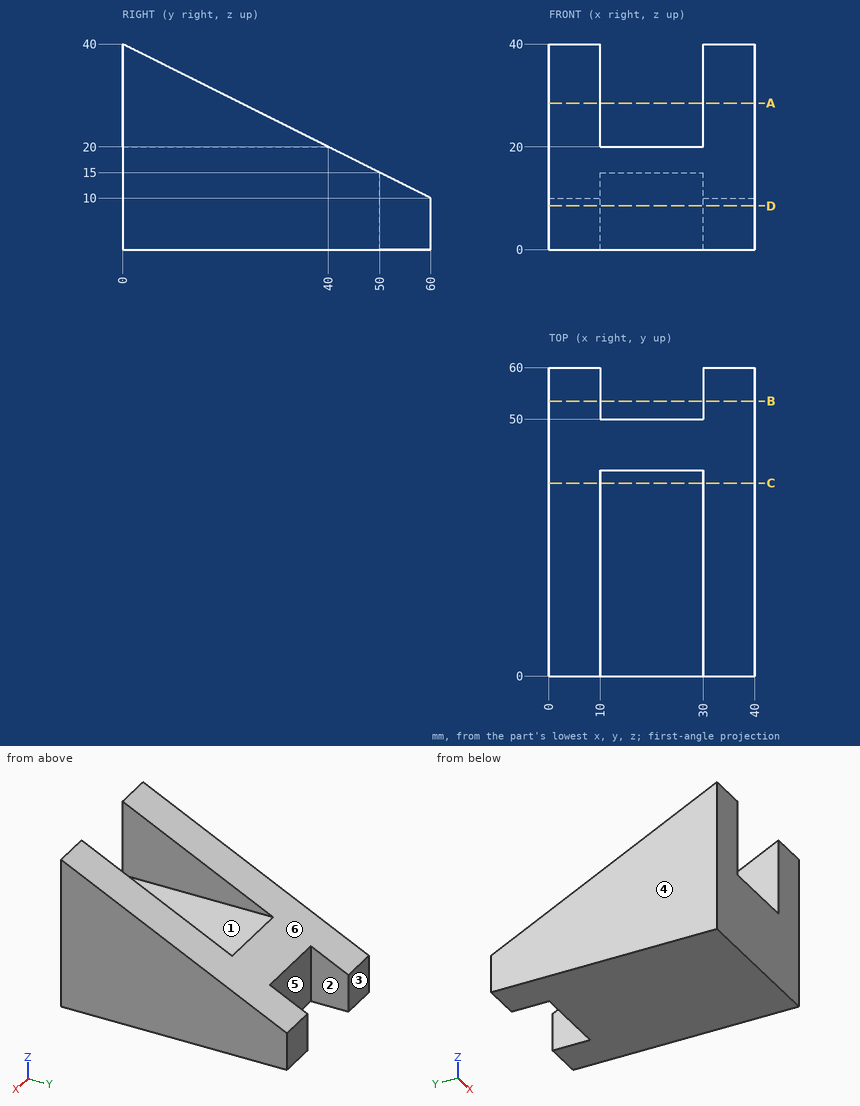
Part print with two shaded views. Sizes in mm from the minimum x, y, z corner. A direction names the side the tool comes from. Coordinates: 2 decimals unless noted, no trailing zeros. Order: outer loops, then holes, each group sorted by start corner. A loop starts at its lowest first (then second) coordinate and runs counter-clockwise, first axis right, second up.
(1) Saw through at D-D, the plane z = 8.5. Write the cut outline in (x, y), and give its area (3 significant figures).
Solution:
outline: (0, 0) - (40, 0) - (40, 60) - (30, 60) - (30, 50) - (10, 50) - (10, 60) - (0, 60) - close
area: 2,200 mm2
(2) Saw through at B-B, the plane y = 53.5. Write the cut outline in (x, z).
Solution:
outline: (0, 0) - (10, 0) - (10, 13.25) - (0, 13.25) - close; (30, 0) - (40, 0) - (40, 13.25) - (30, 13.25) - close
(3) Saw through at A-A, the plane z = 28.5. Write the cut outline in (x, y), and give its area (3 significant figures).
Solution:
outline: (0, 0) - (10, 0) - (10, 23) - (0, 23) - close; (30, 0) - (40, 0) - (40, 23) - (30, 23) - close
area: 460 mm2
(4) Which spindle directions (+Z, -Z, +X, -X, +Y, -Y) get a long thin tool onto all of the face, cutting with end or side? Do the marked faces 1, 2 and 3. Say none if no direction does.
Solution:
face 1: +Z, +Y, -Y
face 2: +Z, -Z, +Y
face 3: +Z, -Z, +X, -X, +Y
(5) Pin check, flat tips, straight feed: pin 1 Ø5 at (y, z) = (28.5, 22.5) entering from -X; pin 2 Ø8 at (x, y) = (23.5, 36.5) entering from +Z; pin 3 Ø5 at (x, y) = (11, 40) entering from +Z; pin 4 Ø2 at (x, z) = (12.5, 13) entering from +Y. Stop position of each tip, or through.
Solution:
pin 1: stops at x = 0
pin 2: stops at z = 20
pin 3: stops at z = 21.15
pin 4: stops at y = 50
(6) Drill centre lines: L1, parallel to X at y = 25, z = 26.5; L2, parallel to Y at x = 12.5, z = 11; L3, parallel to Y at x = 34, z = 30. Where is each one in solid material? Low to high.
Solution:
L1: x = 0 to 10, 30 to 40
L2: y = 0 to 50
L3: y = 0 to 20
(7) Saw through at C-C, the plane y = 37.5. Write the cut outline in (x, z), and give its area (3 significant figures).
Solution:
outline: (0, 0) - (40, 0) - (40, 21.25) - (30, 21.25) - (30, 20) - (10, 20) - (10, 21.25) - (0, 21.25) - close
area: 825 mm2
(8) Mould opens along X. For the marked faces 4, 5 and 6 say: released by +X, released by -X, zero draft, split by the parting line, or undercut.
Solution:
face 4: released by -X
face 5: undercut
face 6: zero draft
